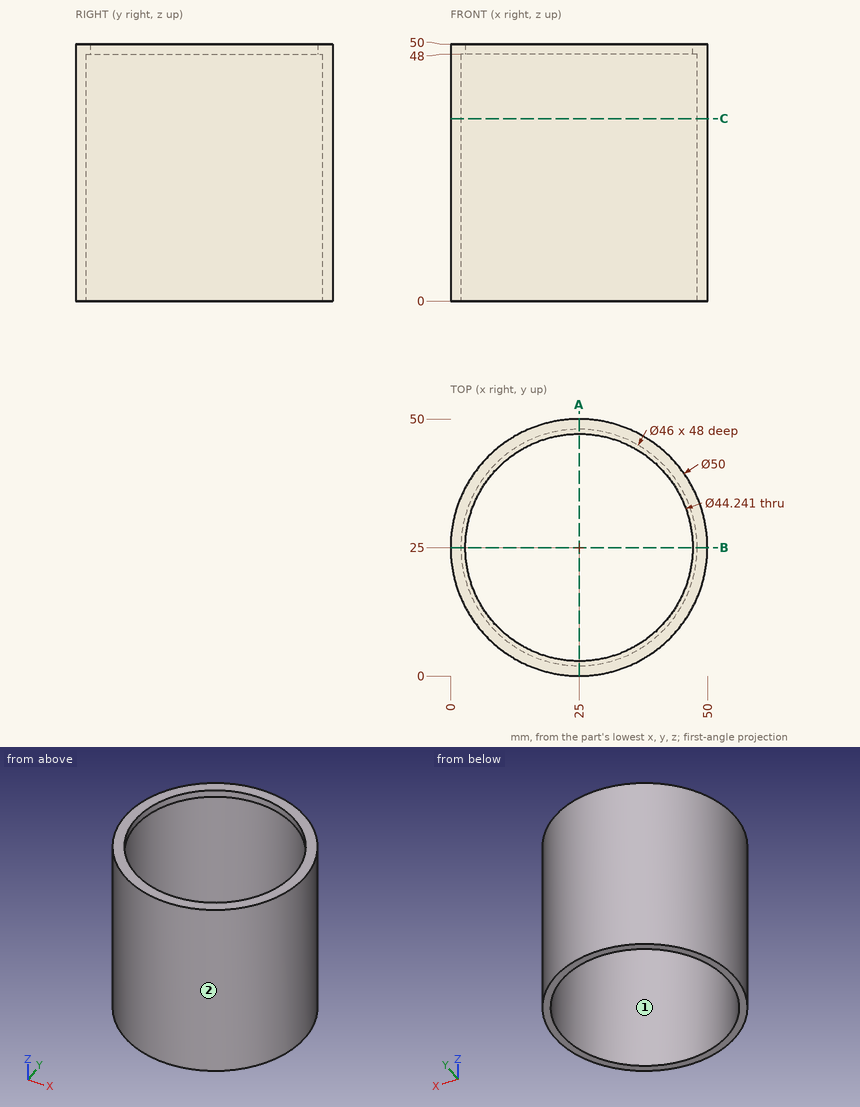
Geometry check sheet. Reference: drawing and pictorial views, mm from the part's lowest x, y, z. Round coordinates to 2 decimals unless told otherwise and drop trailing zeros. Order: outer loops, then holes, each group sorted by start corner. A loop starts at its lowest first (then second) coordinate and runs counter-clockwise, first axis right, second up. Notation, with made-up numbers: (23.5, -6) - (50.5, -6) arc R10 cw to (50.5, 7) - close; hole circle Ø1 at (-31, -7). An arc over 180 degrees is marked (long way). Write item = value, one per line.
Q1. Section check A-A (x = 25). Record the boundary of the cut face in (y, z).
Computed:
outline = (0, 0) - (2, 0) - (2, 48) - (2.88, 48) - (2.88, 50) - (0, 50) - close; (47.12, 48) - (48, 48) - (48, 0) - (50, 0) - (50, 50) - (47.12, 50) - close
Q2. Thickness scan on line 1 along Y through (x, z) = (25, 31); line 2 along X through (y, z) = (16, 25); line 3 along Y through (x, z) = (17.5, 34). Record the ranges inside material, lowest first.
Computed:
line_1 = 0 to 2, 48 to 50
line_2 = 1.68 to 3.83, 46.17 to 48.32
line_3 = 1.15 to 3.26, 46.74 to 48.85
Q3. Go/stop test with flat-tipped pins: pin 1 (1.5 mm diameter, centred on y = 18.5, z = 43.5, fed in from +X); pin 2 (1 mm diameter, centred on x = 28.5, z = 34.5, fed in from +Y); pin 3 (6 mm diameter, centred on x = 25, z = 14, fed in from -Y). Record where each tip stops, or that it passes through.
Computed:
pin_1 = 49.33
pin_2 = 49.82
pin_3 = 0
Q4. Draft check along X on the marked faces 1 and 2. Enter one of: pulls with the +X half, pulls with the -X half, needs draft (parallel to the pull), parting line crosses it, or undercut.
Computed:
face_1 = undercut
face_2 = parting line crosses it
Q5. Section check C-C (z = 35.5). Record the boundary of the cut face in (x, y).
Computed:
outline = circle Ø50 at (25, 25); hole circle Ø46 at (25, 25)
